Autodesk Inventor part; units mm, degrees
ref_plane "Work Plane1" through (0, 9, 0) normal (0, 1, 0) x (-1, 0, 0)
ref_plane "Work Plane2" through (0, 0, 11) normal (0, 0, -1) x (-1, 0, 0)
ref_plane "Work Plane3" through (0, 0, 51) normal (0, 0, 1) x (1, 0, 0)
sketch "Sketch1" plane through (0, 0, 0) normal (0, 0, 1) x (1, 0, 0)
  arc A0 (-1.5, -1.3229) -> (-1.5, 1.3229) centre (0, 0) ccw
  line L0 (-1.5, 1.3229) -> (-1.5, -1.3229)
  circle A1 centre (0, 0) radius 5
  dimension "d0" = 4
  dimension "d2" = 10
extrude "Extrusion1" add sketch "Sketch1" along normal blind 8
sketch "Sketch2" plane through (0, 0, 8) normal (0, 0, 1) x (1, 0, 0)
  point P0 (0, 0)
sketch "Sketch3" plane through (0, 0, 8) normal (0, 0, 1) x (1, 0, 0)
  circle A0 centre (0, 0) radius 7
  dimension "d5" = 14
extrude "Extrusion2" add sketch "Sketch3" along normal blind 35
ref_plane "Work Plane1" through (0, 9, 0) normal (0, 1, 0) x (-1, 0, 0)
sketch "Sketch4" plane through (0, 9, 0) normal (0, 1, 0) x (-1, 0, 0)
  line L0 (0, 20.5) -> (0, 20.5)
  line L1 (-2, 22.5) -> (-2, 36.5)
  line L2 (0, 38.5) -> (0, 38.5)
  line L3 (2, 36.5) -> (2, 22.5)
  line L4 (0, -7.7828) -> (0, 46.6971)
  line L5 (7, 8) -> (-7, 8)
  arc A0 (0, 20.5) -> (2, 22.5) centre (0, 22.5) ccw
  arc A1 (-2, 22.5) -> (0, 20.5) centre (0, 22.5) ccw
  arc A2 (2, 36.5) -> (0, 38.5) centre (0, 36.5) ccw
  arc A3 (0, 38.5) -> (-2, 36.5) centre (0, 36.5) ccw
  line L6 (4.0307, 31) -> (-5.3749, 31) construction
  point P0 (0, 0)
  point P1 (-2, 38.5)
  point P2 (-2, 20.5)
  point P3 (2, 38.5)
  point P4 (0, 38.5)
  point P5 (0, 20.5)
  point P6 (0, 38.5)
  point P7 (0, 20.5)
  point P8 (0, 20.5)
  point P9 (0, 38.5)
  dimension "d9" = 18
  dimension "d10" = 4
  dimension "d11" = 12.5
  dimension "d12" = 2
extrude "Extrusion3" add sketch "Sketch4" against normal up to surface
sketch "Sketch5" plane through (0, 0, 8) normal (0, 0, -1) x (-1, 0, 0)
  circle A0 centre (0, 0) radius 6
  circle A1 centre (0, 0) radius 7
  dimension "d15" = 12
extrude "Extrusion4" cut sketch "Sketch5" against normal blind 11
sketch "Sketch6" plane through (0, 0, 43) normal (0, 0, 1) x (1, 0, 0)
  arc A0 (-1.5, -1.3229) -> (-1.5, 1.3229) centre (0, 0) ccw
  circle A1 centre (0, 0) radius 6
  dimension "d18" = 12
extrude "Extrusion5" add sketch "Sketch6" along normal blind 11
ref_plane "Work Plane2" through (0, 0, 11) normal (0, 0, -1) x (-1, 0, 0)
ref_plane "Work Plane3" through (0, 0, 51) normal (0, 0, 1) x (1, 0, 0)
sketch "Sketch8" plane through (0, 0, 51) normal (0, 0, 1) x (1, 0, 0)
  circle A0 centre (0, 0) radius 5.75
  arc A1 (-1.5, -1.3229) -> (-1.5, 1.3229) centre (0, 0) ccw
  circle A2 centre (0, 0) radius 6
  dimension "d27" = 11.5
  dimension "d28" = 12
extrude "Extrusion7" cut sketch "Sketch8" along normal blind 1.2
sketch "Sketch9" plane through (0, 0, 0) normal (0, 0, -1) x (-1, 0, 0)
  circle A0 centre (0, 0) radius 5
  line L0 (1.5, -1.3229) -> (1.5, 1.3229)
  arc A1 (1.5, 1.3229) -> (1.5, -1.3229) centre (0, 0) ccw
extrude "Extrusion8" cut sketch "Sketch9" against normal blind 2.5
sketch "Sketch10" plane through (0, 0, 8) normal (0, 0, -1) x (-1, 0, 0)
  arc A0 (1.5, 1.3229) -> (1.5, -1.3229) centre (0, 0) ccw
  line L0 (1.5, -1.3229) -> (1.5, 1.3229)
extrude "Extrusion9" cut sketch "Sketch10" against normal blind 2.7
sketch "Sketch11" plane through (0, 0, 8) normal (0, 0, -1) x (-1, 0, 0)
  line L0 (1.5, 1.3229) -> (1.5, -1.3229)
  arc A0 (1.5, 1.3229) -> (1.5, -1.3229) centre (0, 0) ccw
extrude "Extrusion10" add sketch "Sketch11" along normal up to surface (5.5 mm away)
sketch "Sketch12" plane through (0, 0, 2.5) normal (0, 0, -1) x (-1, 0, 0)
  circle A0 centre (0, 0) radius 1.5
  line L0 (-2.5408, -1.5951) -> (-2.4576, 1.7205)
  arc A1 (-2.5408, -1.5951) -> (-2.4576, 1.7205) centre (0, 0) ccw
  point P0 (0, 0)
extrude "Extrusion11" cut sketch "Sketch12" against normal blind 12 contours A0 | L0 A1
properties part number "shatft extension"
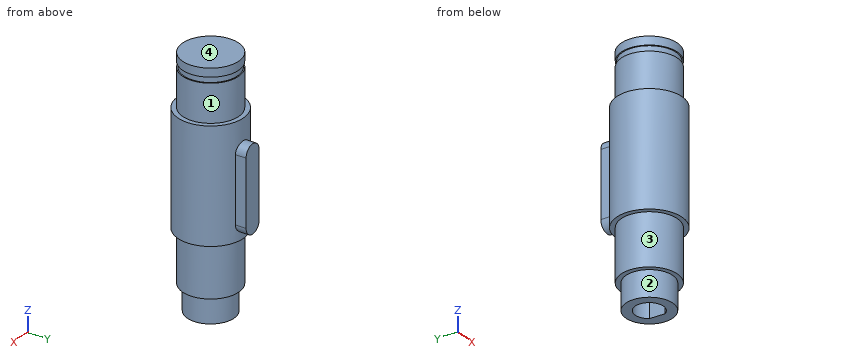
Source: CAD feature listing. Evaluate the final solid. Frame: model axes, mm. Face numbers are marked on the shaded views. A direction names the side the tool comes from. Coordinates: 2 decimals unless noted, no trailing zeros. Order: outer loops, then holes, each group sorted by start corner. A loop starts at its lowest first (then second) coordinate and runs counter-clockwise, first axis right, second up.
Item 1: Set-up query: the marked faces 1 and 2. Return all of +Z, -Z, +X, -X, +Y, -Y with unobstructed straight access to the full face (end or side cutting, diameter ignored); none if empty.
Output values:
face 1: +Z
face 2: -Z
Item 2: Cut plane B-B (y = -2.5). Return loops of the section in (x, z), plus the area to 3 significant figures.
Output values:
outline: (-6.54, 19) - (-5.45, 19) - (-5.45, 8) - (-4.33, 8) - (-4.33, 2.5) - (-1.66, 2.5) - (-1.66, 14.5) - (1.66, 14.5) - (1.66, 2.5) - (4.33, 2.5) - (4.33, 8) - (5.45, 8) - (5.45, 19) - (6.54, 19) - (6.54, 43) - (5.45, 43) - (5.45, 51) - (5.18, 51) - (5.18, 52.2) - (5.45, 52.2) - (5.45, 54) - (-5.45, 54) - (-5.45, 52.2) - (-5.18, 52.2) - (-5.18, 51) - (-5.45, 51) - (-5.45, 43) - (-6.54, 43) - close
area: 561 mm2
Item 3: Material intervals for line 1 (X direction, y = 7.75, z = 29); line 2 (X direction, y = -1.25, z = 6); line 3 (Z direction, x = 0.75, y = 2.5), sorted ascending.
Output values:
line 1: x = -2 to 2
line 2: x = -4.84 to -2.73, 2.53 to 4.84
line 3: z = 14.5 to 54
Item 4: Pull-direction query (Y, two-part tool) for the marked faces 3 and 4; classes: pulls with the +Y half, pulls with the -Y half, needs draft (parallel to the pull), parting line crosses it, or undercut.
Output values:
face 3: parting line crosses it
face 4: needs draft
Item 5: Cut plane C-C (z = 42). Return loops of the section in (x, y), plus the area to 3 significant figures.
Output values:
outline: circle Ø14 at (0, 0)
area: 154 mm2
Item 6: First-contact query: P1, Ø6, axis at x = -4, z = 47, coming from the +Y side; P2, Ø4, axis at x = 0.5, z = 12, coming from the -Y side; P3, Ø2.5, axis at y = 7.5, z = 31.5, coming from the +X side. Flat tips, straight axial feed; report the tip coordinate or a pass-through.
Output values:
P1: stops at y = 5.92
P2: stops at y = -6
P3: stops at x = 3.15
Item 7: Cut plane D-D (y = 7.5). Return loops of the section in (x, z), plus the area to 3 significant figures.
Output values:
outline: (-2, 22.5) arc R2 ccw to (2, 22.5) - (2, 36.5) arc R2 ccw to (-2, 36.5) - close
area: 68.6 mm2
